Part model, mm, in its own coordinate system. Face numbers are marked on the shaded views. A direction names the side the tool comes from. Coordinates: 2 decimals unless noted, no trailing zeros. Order: outer loops, then holes, each group sorted by start corner. A loop starts at its lowest first (then second) coordinate and runs counter-clockwise, first axis right, second up.
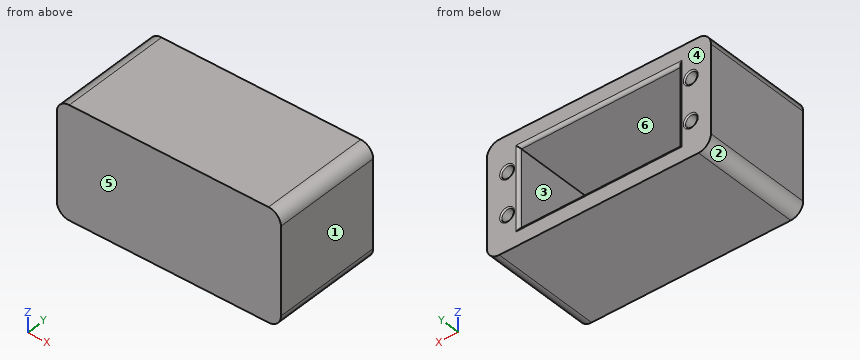
```python
from build123d import *

# Parameters (mm, degrees)
SKETCH1_W           = 91.44
SKETCH1_H           = 45.72
BOSS_EXTRUDE1_DEPTH = 45
SKETCH2_W           = 65.278
SKETCH2_H           = 31.75
CUT_EXTRUDE1_DEPTH  = 40
SKETCH3_R           = 2.5
CUT_EXTRUDE2_DEPTH  = 25.4
FILLET1_R           = 5.08
FILLET3_R           = 1.27
FILLET4_R           = 0.508


with BuildPart() as part:
    # Sketch1 → Boss-Extrude1 (new body)
    with BuildSketch(Plane(origin=(0, 0, 0), x_dir=(1, 0, 0), z_dir=(0, 1, 0))):
        Rectangle(SKETCH1_W, SKETCH1_H)
    extrude(amount=BOSS_EXTRUDE1_DEPTH)

    # Sketch2 → Cut-Extrude1 (cut)
    with BuildSketch(Plane(origin=(0, 45, 0), x_dir=(1, 0, 0), z_dir=(0, 1, 0))):
        Rectangle(SKETCH2_W, SKETCH2_H)
    extrude(amount=-CUT_EXTRUDE1_DEPTH, mode=Mode.SUBTRACT)

    # Sketch3 → Cut-Extrude2 (cut)
    with BuildSketch(Plane(origin=(0, 45, 0), x_dir=(1, 0, 0), z_dir=(0, 1, 0))):
        with Locations(Location((37.465, 8.509, 0), (0, 0, 270))):
            Circle(SKETCH3_R)
        with Locations(Location((37.465, -8.509, 0), (0, 0, 270))):
            Circle(SKETCH3_R)
        with Locations(Location((-37.465, -8.509, 0), (0, 0, 90))):
            Circle(SKETCH3_R)
        with Locations(Location((-37.465, 8.509, 0), (0, 0, 90))):
            Circle(SKETCH3_R)
    extrude(amount=-CUT_EXTRUDE2_DEPTH, mode=Mode.SUBTRACT)

    # Fillet1
    fillet1_edges = [part.edges().sort_by_distance(p)[0] for p in [
        (45.72, 22.5, 22.86),
        (-45.72, 22.5, 22.86),
        (-45.72, 22.5, -22.86),
        (45.72, 22.5, -22.86),
    ]]
    fillet(fillet1_edges, radius=FILLET1_R)

    # Fillet3
    fillet3_edges = [part.edges().sort_by_distance(p)[0] for p in [
        (32.639, 45, 0),
        (0, 45, -15.875),
        (-32.639, 45, 0),
        (0, 45, 15.875),
    ]]
    fillet(fillet3_edges, radius=FILLET3_R)

    # Fillet4
    fillet4_edges = [part.edges().sort_by_distance(p)[0] for p in [
        (-37.465, 45, -6.009),
        (-37.465, 45, 11.009),
        (37.465, 45, 6.009),
        (37.465, 45, -11.009),
    ]]
    fillet(fillet4_edges, radius=FILLET4_R)


solid = part.part
```
(1) Probe line 1 (X direction, y = 15, z = -1); line 2 (X direction, y = 40, z = -8.5); line 3 (Z direction, x = -10, y = 19) (3 decimals). List the from-to ranges inside material, lowest first.
(2) Slice it at A-A, the plane x = 0. Give the cut face in (y, z) (3 decimals), then the cut area to 3 significant figures.
(3) Pull direction X, two halves, no side cores. Call the marked faces 1, 2, 3 and 4: +X half, -X half, draft (parallel to the pull), parting line (faces both ways), or undercut.
(4) Slice it at B-B, the plane z = -14.5. Give the cut face in (x, y).
(5) Drop flat-ended pins along their axis: pin 1 (2.5 mm diameter, centred on x = -38, z = 9, fed in from +Y); pin 2 (8 mm diameter, centred on x = 16, z = -10, fed in from +Y). Give the stop position or say it passes through.
(6) Slice it at C-C, the plane y = 29. Give the cut face in (x, z) (3 decimals).
(7) Tool access for the marked faces 5 and 6: list every direction of +Z, -Z, +X, -X, +Y, -Y with a clear straight run to the whole face (end or side of a thin tool).
Here are the results:
1. line 1: x = -45.72 to -32.64, 32.64 to 45.72
1. line 2: x = -45.72 to -39.96, -34.97 to -32.64, 32.64 to 34.97, 39.96 to 45.72
1. line 3: z = -22.86 to -15.875, 15.875 to 22.86
2. outline: (0, -22.86) - (45, -22.86) - (45, -17.145) arc R1.27 ccw to (43.73, -15.875) - (5, -15.875) - (5, 15.875) - (43.73, 15.875) arc R1.27 ccw to (45, 17.145) - (45, 22.86) - (0, 22.86) - close
2. area: 787 mm2
3. face 1: +X half
3. face 2: -X half
3. face 3: undercut
3. face 4: draft
4. outline: (-45.72, 0) - (45.72, 0) - (45.72, 45) - (33.91, 45) arc R1.27 ccw to (32.64, 43.73) - (32.64, 5) - (-32.64, 5) - (-32.64, 43.73) arc R1.27 ccw to (-33.91, 45) - (-45.72, 45) - close
5. pin 1: stops at y = 19.6
5. pin 2: stops at y = 5
6. outline: (-45.72, -17.78) arc R5.08 ccw to (-40.64, -22.86) - (40.64, -22.86) arc R5.08 ccw to (45.72, -17.78) - (45.72, 17.78) arc R5.08 ccw to (40.64, 22.86) - (-40.64, 22.86) arc R5.08 ccw to (-45.72, 17.78) - close; hole circle Ø5 at (-37.465, -8.509); hole circle Ø5 at (-37.465, 8.509); hole (-32.639, -15.875) - (32.639, -15.875) - (32.639, 15.875) - (-32.639, 15.875) - close; hole circle Ø5 at (37.465, -8.509); hole circle Ø5 at (37.465, 8.509)
7. face 5: +Z, -Z, +X, -X, -Y
7. face 6: +Y
